Autodesk Inventor part; units mm, degrees
ref_plane "Work Plane1" through (-47.403, 13.795, 36.5962) normal (0, 1, 0) x (1, 0, 0)
ref_plane "YZ Plane" through (0, 0, 0) normal (1, 0, 0) x (0, 1, 0)
ref_plane "XZ Plane" through (0, 0, 0) normal (0, 1, 0) x (-1, 0, 0)
sketch "Sketch1" plane through (0, 0, 0) normal (0, 1, 0) x (-1, 0, 0)
  line L0 (-2.922, 0) -> (47.078, 0)
  line L1 (47.078, 0) -> (47.078, 33.0962)
  line L2 (47.078, 33.0962) -> (-2.922, 33.0962)
  line L3 (-2.922, 33.0962) -> (-2.922, 0)
  line L4 (50.578, 36.5962) -> (50.578, -3.5)
  line L5 (50.578, -3.5) -> (-6.422, -3.5)
  line L6 (-6.422, -3.5) -> (-6.422, 36.5962)
  line L7 (-6.422, 36.5962) -> (50.578, 36.5962)
  point P0 (0, 0)
  dimension "d0" = 50
  dimension "d1" = 33.0962
  dimension "d2" = 3.5
extrude "Extrusion1" add sketch "Sketch1" along normal blind 13.97 contours L3 L2 L1 L0 | L4 L5 L6 L7
shell "Shell1" thickness 3 removed faces 0
sketch "Sketch2" plane through (0, 13.97, 0) normal (0, 1, 0) x (1, 0, 0)
  point P0 (0, 0)
move faces "Move1" translate (0, -3.175, 0) faces at (-12.578, 13.97, 23.2308)
move faces "Move2" translate (0, 3, 0) faces at (-13.578, 10.795, 35.5962)
fillet "Fillet1" radius 3.175 4 edges at (6.422, 6.8975, 36.5962) (6.422, 6.8975, -3.5) (-50.578, 6.8975, -3.5) (-50.578, 6.8975, 36.5962)
ref_plane "Work Plane1" through (-47.403, 13.795, 36.5962) normal (0, 1, 0) x (1, 0, 0)
sketch "Sketch3" plane through (-47.403, 13.795, 36.5962) normal (0, 1, 0) x (1, 0, 0)
  arc A0 (-3.175, 3.175) -> (0, 0) centre (0, 3.175) ccw
  line L0 (0, 0) -> (50.65, 0)
  arc A1 (50.65, 0) -> (53.825, 3.175) centre (50.65, 3.175) ccw
  line L1 (53.825, 3.175) -> (53.825, 36.9212)
  arc A2 (53.825, 36.9212) -> (50.65, 40.0962) centre (50.65, 36.9212) ccw
  line L2 (50.65, 40.0962) -> (0, 40.0962)
  arc A3 (0, 40.0962) -> (-3.175, 36.9212) centre (0, 36.9212) ccw
  line L3 (-3.175, 36.9212) -> (-3.175, 3.175)
  line L4 (50.825, 3) -> (-0.175, 3)
  line L5 (-0.175, 3) -> (-0.175, 37.0962)
  line L6 (-0.175, 37.0962) -> (50.825, 37.0962)
  line L7 (50.825, 37.0962) -> (50.825, 3)
  point P0 (47.403, 36.5962)
sketch "Sketch4" plane through (0, 0, 0) normal (0, -1, 0) x (1, 0, 0)
  arc A0 (-50.578, 33.4212) -> (-47.403, 36.5962) centre (-47.403, 33.4212) ccw
  line L0 (-50.578, -0.325) -> (-50.578, 33.4212)
  arc A1 (-47.403, -3.5) -> (-50.578, -0.325) centre (-47.403, -0.325) ccw
  line L1 (3.247, -3.5) -> (-47.403, -3.5)
  arc A2 (6.422, -0.325) -> (3.247, -3.5) centre (3.247, -0.325) ccw
  line L2 (6.422, 33.4212) -> (6.422, -0.325)
  arc A3 (3.247, 36.5962) -> (6.422, 33.4212) centre (3.247, 33.4212) ccw
  line L3 (-47.403, 36.5962) -> (3.247, 36.5962)
  line L4 (-41.4583, 43.9872) -> (-33.9992, 43.9872)
  line L5 (-33.9992, 43.9872) -> (-33.9992, -11.1575)
  line L6 (-33.9992, -11.1575) -> (-41.4583, -11.1575)
  line L7 (-41.4583, -11.1575) -> (-41.4583, 43.9872)
  line L8 (-11.5895, 44.289) -> (-4.1219, 44.289)
  line L9 (-4.1219, 44.289) -> (-4.1219, -11.1575)
  line L10 (-4.1219, -11.1575) -> (-11.5895, -11.1575)
  line L11 (-11.5895, -11.1575) -> (-11.5895, 44.289)
  point P0 (0, 0)
  dimension "d15" = 7.4591
  dimension "d16" = 55.1447
  dimension "d17" = 7.4676
extrude "Extrusion2" add sketch "Sketch4" against normal blind 2.8575 contours L7 L4 L5 L3 | L3 L5 L1 L7 | L1 L5 L6 L7 | L11 L8 L9 L3 | L3 L9 L1 L11 | L1 L9 L10 L11
properties part number "Gyro_box_bottom"
Read the model definition and answer for the solid it produces. Units are mm, in the model's axes. A direction names the side the tool comes from. Coordinates: 2 decimals unless noted, no trailing zeros. Write each loop counter-clockwise with the first axis right and the second up, starting at its lowest first coordinate (ties: lowest second). Pieces come first, ordered by that corner, then holes. Notation, with made-up numbers: (50.5, -39) -> (58.5, -39) arc R35 cw to (58.5, -1) -> close; hole circle Ø7 at (16, -24). An arc over 180 degrees is marked (long way). Return JSON: item names as keys, results as strings.
1. Find the intervals of material crossed by line 1 along X through (y, z) = (13, 3); line 2 along Z through (x, y) = (-27.5, 12.5); line 3 along Z through (x, y) = (-33.5, 1.25), in increasing order. Write a range as from..to.
Found:
{"line 1": "-50.58..-47.58, 3.42..6.42", "line 2": "-3.5..-0.5, 33.6..36.6", "line 3": "-3.5..36.6"}
2. A cutting plane is placed at D-D (x = -6). Determine the outline of the cut face in (y, z) (1 decimal), and give its area (3 significant figures).
Found:
{"outline": "(0, -11.2) -> (2.9, -11.2) -> (2.9, -3.5) -> (13.8, -3.5) -> (13.8, -0.5) -> (3, -0.5) -> (3, 33.6) -> (13.8, 33.6) -> (13.8, 36.6) -> (2.9, 36.6) -> (2.9, 44.3) -> (0, 44.3) -> close", "area": "229 mm2"}
3. Determine the mould class of faces 1 (the face through (-11.59, 1, 40)), 2 (the face through (-4.122, 1, 40)), 3 (the face through (-41.458, 1, -7)) for opening direction X: pulls with the +X half, pulls with the -X half, needs draft (parallel to the pull), parting line crosses it, or undercut.
Found:
{"face 1": "undercut", "face 2": "pulls with the +X half", "face 3": "pulls with the -X half"}
4. A cutting plane is placed at A-A (y = 11.5). Determine the outline of the cut face in (x, z) (3 decimals).
Found:
{"outline": "(-50.578, -0.325) arc R3.175 ccw to (-47.403, -3.5) -> (3.247, -3.5) arc R3.175 ccw to (6.422, -0.325) -> (6.422, 33.421) arc R3.175 ccw to (3.247, 36.596) -> (-47.403, 36.596) arc R3.175 ccw to (-50.578, 33.421) -> close; hole (-47.578, -0.5) -> (3.422, -0.5) -> (3.422, 33.596) -> (-47.578, 33.596) -> close"}
5. A tool of negligible diameter and unlimited length cuts with its end or side. For faces 4 (the face through (-33.999, 1, 40)), 5 (the face through (-8, 2.858, -7)), 6 (the face through (-8, 2.858, 40)), from which of +Z, -Z, +X, -X, +Y, -Y can it reach the whole face along a straight path? Write none if from no direction.
Found:
{"face 4": "+Z, +Y, -Y", "face 5": "-Z, +X, -X, +Y", "face 6": "+Z, +X, -X, +Y"}
6. A cutting plane is placed at B-B (x = -17). Determine the outline of the cut face in (y, z) (3 decimals).
Found:
{"outline": "(0, -3.5) -> (13.795, -3.5) -> (13.795, -0.5) -> (3, -0.5) -> (3, 33.596) -> (13.795, 33.596) -> (13.795, 36.596) -> (0, 36.596) -> close"}
7. Each of these flat-tipped pins is pushed along its axis until it touches: P1, Ø8, axis at x = -36.5, z = 42, coming from the +Y side; P2, Ø1.4, axis at y = 1, z = 39, coming from the -X side; P3, Ø3, axis at x = -37.5, y = 2, coming from the +Z side; P4, Ø4, axis at x = -18, z = 14, coming from the -Y side. Where does it stop, or does it pass through?
Found:
{"P1": "y = 2.86", "P2": "x = -41.46", "P3": "z = 43.99", "P4": "y = 0"}
8. A cutting plane is placed at C-C (z = 5). Determine the outline of the cut face in (x, y) (3 decimals), and give its area (3 significant figures).
Found:
{"outline": "(-50.578, 0) -> (6.422, 0) -> (6.422, 13.795) -> (3.422, 13.795) -> (3.422, 3) -> (-47.578, 3) -> (-47.578, 13.795) -> (-50.578, 13.795) -> close", "area": "236 mm2"}
